Read the model definition and answer for the solid it produces. Units are mm, in the model's axes. Round coordinates to 2 decimals unless told otherwise and drop trailing zeros. Loops run counter-clockwise (first coordinate to the right, second up) from the corner with the lowest first, then second, coordinate; pieces in that order, holes last. Notation, with made-up numbers: M 31,4.5 L 40,4.5 A18 cw 40,33.5 Z; hole C 30,86.25 d11. An arc over 180 degrees is marked long. Write each question's results on one line, items separated by ' | '.
```python
from build123d import *

# Parameters (mm, degrees)
SKETCH1_W           = 19
SKETCH1_H           = 19
BOSS_EXTRUDE1_DEPTH = 19
SKETCH2_R           = 4.75
CUT_EXTRUDE1_DEPTH  = 19
SKETCH3_R           = 4.75
CUT_EXTRUDE2_DEPTH  = 19


with BuildPart() as part:
    # Sketch1 → Boss-Extrude1 (new body)
    with BuildSketch(Plane(origin=(0, 0, 0), x_dir=(1, 0, 0), z_dir=(0, 1, 0))):
        with Locations((9.5, 9.5)):
            Rectangle(SKETCH1_W, SKETCH1_H)
    extrude(amount=BOSS_EXTRUDE1_DEPTH)

    # Sketch2 → Cut-Extrude1 (cut)
    with BuildSketch(Plane(origin=(0, 19, 0), x_dir=(1, 0, 0), z_dir=(0, 1, 0))):
        with Locations((9.5, 9.5)):
            Circle(SKETCH2_R)
    extrude(amount=-CUT_EXTRUDE1_DEPTH, mode=Mode.SUBTRACT)

    # Sketch3 → Cut-Extrude2 (cut)
    with BuildSketch(Plane.XY):
        with Locations((9.5, 9.5)):
            Circle(SKETCH3_R)
    extrude(amount=-CUT_EXTRUDE2_DEPTH, mode=Mode.SUBTRACT)


solid = part.part
```
1. Find section D-D, the plane z = -6.75. Give the vertices of the cut face in (x, y), then the cut area to 3 significant figures.
Completed:
outline: M 0,0 L 5.63,0 L 5.63,6.75 A4.75 cw 5.63,12.25 L 5.63,19 L 0,19 Z; M 13.37,0 L 19,0 L 19,19 L 13.37,19 L 13.37,12.25 A4.75 cw 13.37,6.75 Z | area: 207 mm2
2. Find section A-A, the plane x = 9.5. Give the vertices of the cut face in (y, z), then the cut area to 4 significant figures.
Completed:
outline: M 0,-19 L 4.75,-19 L 4.75,-14.25 L 0,-14.25 Z; M 0,-4.75 L 4.75,-4.75 L 4.75,0 L 0,0 Z; M 14.25,-19 L 19,-19 L 19,-14.25 L 14.25,-14.25 Z; M 14.25,-4.75 L 19,-4.75 L 19,0 L 14.25,0 Z | area: 90.25 mm2
3. Determine the mould class of faces 1 (the face through (19, 9, -9)), 2 (the face through (6, 12.71, -3.63)), 3 (the face through (5, 0, -12)) for opening direction X: released by +X, released by -X, zero draft, split by the parting line, or undercut.
Completed:
face 1: released by +X | face 2: undercut | face 3: zero draft
4. Find section C-C, the plane y = 11.75. Give the vertices of the cut face in (x, z), then the cut area to 3 significant figures.
Completed:
outline: M 0,-19 L 5.32,-19 L 5.32,-11.75 A4.75 cw 5.32,-7.25 L 5.32,0 L 0,0 Z; M 13.68,-19 L 19,-19 L 19,0 L 13.68,0 L 13.68,-7.25 A4.75 cw 13.68,-11.75 Z | area: 199 mm2
5. Given P1, Ø7.5, axis at x = 9.5, z = -9.5, coming from the -Y side; P2, Ø1, axis at x = 10.5, y = 16, coming from the +Z side, each flat-ended and moving along its own axis, determine where each tip first touches the part or whether it passes through.
Completed:
P1: passes through | P2: stops at z = 0
6. Find section B-B, the plane z = -3. Give the vertices of the cut face in (x, y), then the cut area to 3 significant figures.
Completed:
outline: M 0,0 L 19,0 L 19,19 L 0,19 Z; hole C 9.5,9.5 d9.5 | area: 290 mm2
7. Find the intervals of material crossed by L1, parallel to X at y = 4.5, z = -9.5; L2, parallel to Z at x = 9.5, y = 4.5, in increasing order.
Completed:
L1: x = 0 to 4.75, 14.25 to 19 | L2: z = -19 to -14.25, -4.75 to 0
